Can you work these out from the model? Positions are in its coordinate system, mm. A direction names the side the tool comes from. Give positions to 0.01 mm unless a question says otherwise; leave off trailing zeros. Loops run counter-clockwise (first coordinate to the right, second up) from the corner with the lowest first, then second, coordinate; pieces in that order, holes last. Notation, with made-up numbers: (-30, 66.5) -> (5, 66.5) arc R12 ccw to (5, 76.5) -> close; hole circle Ø2 at (63.5, -20). An arc over 180 degrees is marked (long way). One line per question, with ' | ' between items.
from build123d import *

# Parameters (mm, degrees)
SKETCH3_W           = 140.715997696
SKETCH3_H           = 60.070999146
SKETCH3_R           = 2.286
SKETCH3_W_2         = 38.1
SKETCH3_H_2         = 12.7
SKETCH3_H_3         = 12.548758089
SKETCH3_H_4         = 22.298299906
BOSS_EXTRUDE1_DEPTH = 3.175
SKETCH4_W           = 38.1
SKETCH4_H           = 9.598299906
BOSS_EXTRUDE2_DEPTH = 1.5875


with BuildPart() as part:
    # Sketch3 → Boss-Extrude1 (new body)
    with BuildSketch(Plane(origin=(0, 0, 0), x_dir=(1, 0, 0), z_dir=(0, 1, 0))):
        with Locations((0.695262938, 7.925997488)):
            Rectangle(SKETCH3_W, SKETCH3_H)
        with Locations((65.211264471, -16.521503733)):
            Circle(SKETCH3_R, mode=Mode.SUBTRACT)
        with Locations((45.270791396, -4.068621014)):
            Rectangle(SKETCH3_W_2, SKETCH3_H_2, mode=Mode.SUBTRACT)
        with Locations((45.270791396, 15.743378986)):
            Rectangle(SKETCH3_W_2, SKETCH3_H_2, mode=Mode.SUBTRACT)
        with Locations((0.820791396, -4.14424197)):
            Rectangle(SKETCH3_W_2, SKETCH3_H_3, mode=Mode.SUBTRACT)
        with Locations((0.820791396, 20.542528939)):
            Rectangle(SKETCH3_W_2, SKETCH3_H_4, mode=Mode.SUBTRACT)
        with Locations((-63.820735529, -16.521503733)):
            Circle(SKETCH3_R, mode=Mode.SUBTRACT)
        with Locations((-43.629208604, -4.068621014)):
            Rectangle(SKETCH3_W_2, SKETCH3_H_2, mode=Mode.SUBTRACT)
        with Locations((-43.629208604, 15.743378986)):
            Rectangle(SKETCH3_W_2, SKETCH3_H_2, mode=Mode.SUBTRACT)
        with Locations((-63.820735529, 31.738496267)):
            Circle(SKETCH3_R, mode=Mode.SUBTRACT)
        with Locations((65.211264471, 31.738496267)):
            Circle(SKETCH3_R, mode=Mode.SUBTRACT)
    extrude(amount=BOSS_EXTRUDE1_DEPTH)

    # Sketch4 → Boss-Extrude2 (add)
    with BuildSketch(Plane(origin=(0, 3.175, 0), x_dir=(1, 0, 0), z_dir=(0, 1, 0))):
        with Locations((0.820791396, 26.892528939)):
            Rectangle(SKETCH4_W, SKETCH4_H)
    extrude(amount=-BOSS_EXTRUDE2_DEPTH)


solid = part.part
Q1. If we section it at A-A (x = 4): Write out the boundary of the cut face in (y, z) (1 decimal), plus the area to 3 significant figures.
Entries:
outline: (0, -38) -> (3.2, -38) -> (3.2, -22.1) -> (1.6, -22.1) -> (1.6, -31.7) -> (0, -31.7) -> close; (0, -9.4) -> (3.2, -9.4) -> (3.2, -2.1) -> (0, -2.1) -> close; (0, 10.4) -> (3.2, 10.4) -> (3.2, 22.1) -> (0, 22.1) -> close | area: 95.3 mm²
Q2. If we section it at B-B (z = -20): Write out the boundary of the cut face in (x, y) (3 decimals), plus the area to 3 significant figures.
Entries:
outline: (-69.663, 0) -> (-62.679, 0) -> (-62.679, 3.175) -> (-69.663, 3.175) -> close; (-24.579, 0) -> (-18.229, 0) -> (-18.229, 3.175) -> (-24.579, 3.175) -> close; (19.871, 0) -> (26.221, 0) -> (26.221, 3.175) -> (19.871, 3.175) -> close; (64.321, 0) -> (71.053, 0) -> (71.053, 3.175) -> (64.321, 3.175) -> close | area: 83.9 mm²
Q3. If we mould it in two halves opening along X, with no side actions, what happens to faces 1 (the face through (-69.663, 2, -8)), 2 (the face through (0, 0, -8)), 3 (the face through (-44, 2, 10.419))? For each: pulls with the +X half, pulls with the -X half, needs draft (parallel to the pull), parting line crosses it, or undercut.
Entries:
face 1: pulls with the -X half | face 2: needs draft | face 3: undercut
Q4. If we section it at D-D (y = 0.55): State how many separate pieces and enclosed holes the cut face has, plus the area to 3 significant figures.
Entries:
separate pieces: 1 | enclosed holes: 10 | area: 5,120 mm²
Q5. If we section it at C-C (x = 29.5): Write out the boundary of the cut face in (y, z) (1 decimal), plus the area to 3 significant figures.
Entries:
outline: (0, -38) -> (3.2, -38) -> (3.2, -22.1) -> (0, -22.1) -> close; (0, -9.4) -> (3.2, -9.4) -> (3.2, -2.3) -> (0, -2.3) -> close; (0, 10.4) -> (3.2, 10.4) -> (3.2, 22.1) -> (0, 22.1) -> close | area: 110 mm²
Q6. On a 3-axis mill with a long thin cutter (end or side, diameter ignored), from which of +Z, -Z, +X, -X, +Y, -Y can I reach the whole of each face in a straight line? I mean faces 4 (the face through (0, 3.175, -8)), 5 (the face through (1, 1.588, -27)), 6 (the face through (19.871, 2, 4)). Say none if no direction works.
Entries:
face 4: +Z, -Z, +X, -X, +Y | face 5: -Y | face 6: +Y, -Y
Q7. For pin 1 Ø8 at (x, z) = (10.5, 6) entering from -Y; pin 2 Ø6 at (x, z) = (-63.82, -31.74) entering from -Y, each with a flat end and sliding along its axis, tell me the tip position at first contact or that it passes through.
Entries:
pin 1: through | pin 2: y = 0
Q8. If I drill on probe 1 along X at (y, z) = (1.2, 6); probe 2 along Z at (x, y) = (-4.5, 0.55); probe 3 along Z at (x, y) = (-60, 0.8), over which ranges is the centre line in solid material (lowest first)? Write a range as from..to.
Entries:
probe 1: -69.66..-62.68, -24.58..-18.23, 19.87..26.22, 64.32..71.05 | probe 2: -37.96..-31.69, -9.39..-2.13, 10.42..22.11 | probe 3: -37.96..-22.09, -9.39..-2.28, 10.42..22.11
